Answer from the drawing. Dimensions are ordinates in mm from the lowest x, y and z of the part. A direction names the side the tool comes from. Coordinates: 2 decimals unless noted, no trailing zeros. Write each loop counter-clockwise with the first axis right and the second up, starting at its lowest first coordinate (ties: lowest second). Pieces come first, ordered by that corner, then holes. Notation, with made-up numbers: (49, -28) -> (70, -28) arc R21 cw to (70, -21) -> close; hole circle Ø9 at (75, 44.25). An arc over 180 degrees is marked (long way). Return JSON: item names as keys, results as strings.
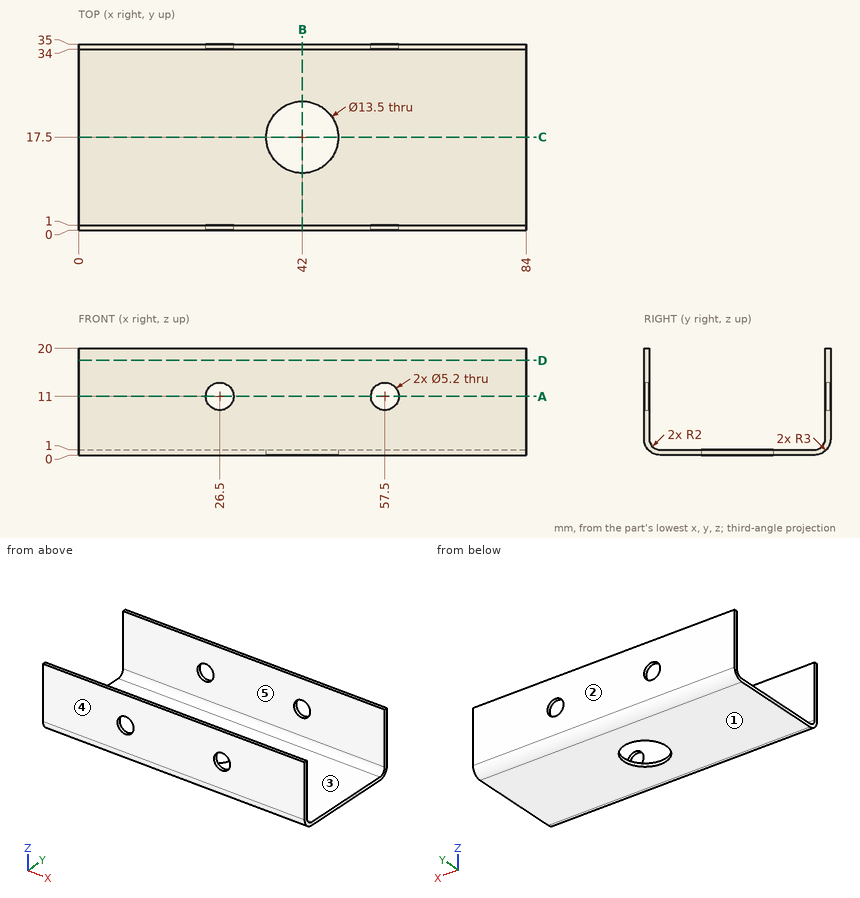
1. A tool of negligible diameter and unlimited length cuts with its end or side. For the marked faces 4 and 5, from which of +Z, -Z, +X, -X, +Y, -Y can it reach the whole face along a straight path? Write none if from no direction.
Taken from the geometry:
{"face 4": "+Z, -Z, +X, -X, -Y", "face 5": "+Z, +X, -X"}
2. The part is cut by section D-D (z = 17.75). Determine the outline of the cut face in (x, y).
Taken from the geometry:
{"outline": "(0, 0) -> (84, 0) -> (84, 1) -> (0, 1) -> close; (0, 34) -> (84, 34) -> (84, 35) -> (0, 35) -> close"}
3. Consider L1, parallel to X at y = 0.3, z = 11; L2, parallel to Y at x = 60, z = 3.5; L3, parallel to Z at x = 75, y = 22. Determine where each line is inside the solid, lowest interval first.
Taken from the geometry:
{"L1": "x = 0 to 23.9, 29.1 to 54.9, 60.1 to 84", "L2": "y = 0 to 1, 34 to 35", "L3": "z = 0 to 1"}
4. The part is cut by section B-B (x = 42). Determine the outline of the cut face in (y, z), then the cut area to 3 significant figures.
Taken from the geometry:
{"outline": "(0, 3) arc R3 ccw to (3, 0) -> (10.75, 0) -> (10.75, 1) -> (3, 1) arc R2 cw to (1, 3) -> (1, 20) -> (0, 20) -> close; (24.25, 0) -> (32, 0) arc R3 ccw to (35, 3) -> (35, 20) -> (34, 20) -> (34, 3) arc R2 cw to (32, 1) -> (24.25, 1) -> close", "area": "57.4 mm2"}
5. For a pull along Y with two mould halves and no side action, classify the marked faces 1, 2 and 3 as +Y half, -Y half, draft (parallel to the pull), parting line (faces both ways), or undercut.
Taken from the geometry:
{"face 1": "draft", "face 2": "+Y half", "face 3": "undercut"}
6. The part is cut by section A-A (z = 11). Determine the outline of the cut face in (x, y), then the cut area to 3 significant figures.
Taken from the geometry:
{"outline": "(0, 0) -> (23.9, 0) -> (23.9, 1) -> (0, 1) -> close; (0, 34) -> (23.9, 34) -> (23.9, 35) -> (0, 35) -> close; (29.1, 0) -> (54.9, 0) -> (54.9, 1) -> (29.1, 1) -> close; (29.1, 34) -> (54.9, 34) -> (54.9, 35) -> (29.1, 35) -> close; (60.1, 0) -> (84, 0) -> (84, 1) -> (60.1, 1) -> close; (60.1, 34) -> (84, 34) -> (84, 35) -> (60.1, 35) -> close", "area": "147 mm2"}
7. The part is cut by section C-C (y = 17.5). Determine the outline of the cut face in (x, z).
Taken from the geometry:
{"outline": "(0, 0) -> (35.25, 0) -> (35.25, 1) -> (0, 1) -> close; (48.75, 0) -> (84, 0) -> (84, 1) -> (48.75, 1) -> close"}
8. Flat-ended cylindrical pins translate along their axes: pin 1 Ø5 at (x, y) = (75, 7) entering from +Z; pin 2 Ø4.5 at (x, z) = (57.5, 11) entering from -Y. Find the tip coordinate at first contact, or state that the pin passes through.
Taken from the geometry:
{"pin 1": "stops at z = 1", "pin 2": "passes through"}
